from build123d import *

# Parameters (mm, degrees)
SKETCH1_W           = 90
SKETCH1_H           = 90
BOSS_EXTRUDE1_DEPTH = 70
SHELL2_T            = -5
CUT_EXTRUDE1_REACH  = 96.604
SKETCH2_W           = 70
SKETCH2_H           = 24
BOSS_EXTRUDE2_DEPTH = 7
SKETCH5_W           = 8
SKETCH5_H           = 10
CUT_EXTRUDE2_DEPTH  = 10


with BuildPart() as part:
    # Sketch1 → Boss-Extrude1 (new body)
    with BuildSketch(Plane.XY):
        Rectangle(SKETCH1_W, SKETCH1_H)
    extrude(amount=BOSS_EXTRUDE1_DEPTH)

    # Shell2
    shell2_openings = [part.faces().sort_by_distance(p)[0] for p in [
        (0, 0, 0),
    ]]
    offset(amount=SHELL2_T, openings=shell2_openings, kind=Kind.INTERSECTION)

    # Sketch2 → Cut-Extrude1 (cut, up to next)
    with BuildSketch(Plane.XY.offset(70), mode=Mode.PRIVATE) as cut_extrude1_sk1:
        with Locations((0, 20)):
            Rectangle(SKETCH2_W, SKETCH2_H)
    cut_extrude1_tool1 = extrude(cut_extrude1_sk1.sketch, amount=-CUT_EXTRUDE1_REACH, mode=Mode.PRIVATE) & part.part
    add(cut_extrude1_tool1.solids().sort_by_distance((0, 20, 70))[0], mode=Mode.SUBTRACT)

    # Sketch4 → Boss-Extrude2 (add)
    with BuildSketch(Plane(origin=(0, 0, 65), x_dir=(-1, 0, 0), z_dir=(0, 0, -1))):
        Polygon((-40, 38), (-40, 32), (-35, 32), (35, 32), (35, 8), (-35, 8), (-40, 8), (-40, 2), (40, 2), (40, 38), align=None)
    extrude(amount=BOSS_EXTRUDE2_DEPTH)

    # Sketch5 → Cut-Extrude2 (cut)
    with BuildSketch(Plane.XY.offset(70)):
        with Locations((0, -7)):
            Rectangle(SKETCH5_W, SKETCH5_H)
    extrude(amount=-CUT_EXTRUDE2_DEPTH, mode=Mode.SUBTRACT)


solid = part.part
Source: CAD feature listing. Evaluate the final solid. Frame: model axes, mm. A direction names the side the tool comes from. Round coordinates to 2 decimals unless told otherwise and drop trailing zeros. Loops run counter-clockwise (first coordinate to the right, second up) from the corner with the lowest first, then second, coordinate; pieces in that order, holes last. Notation, with made-up numbers: (74, 59) -> (114, 59) arc R13 ccw to (114, 66) -> close; hole circle Ø1 at (88, 24.5). An arc over 180 degrees is marked (long way). Answer as a JSON object with one key per item and string values. Group by question number.
Q1. Section query D-D (x = -2). Output: boundary loops of the cut face in (y, z), plus the area to 3 significant figures.
Q2. Contact query for a flat-ended pin moving along its axis: P1, Ø12.5, axis at x = -18, y = -21.5, coming from the -Z side. Output: stop coordinate, or through.
Q3. Access query for faces 5 (the flat face through (35, 20, 68)), 6 (the flat face through (-1, 40, 32)), 7 (the flat face through (-45, -1, 35)). Directions: +Z, -Z, +X, -X, +Y, -Y. A direction counts if a zero-diameter tool reaches every point of the face in a straight line with its end or side. Return the directions, or none.
Q4. Mould query, pull axis X, two halves, no side actions, for faces 1 (the flat face through (45, -1, 35)), 2 (the flat face through (0, -12, 68)), 3 (the flat face through (-1, 45, 35)), 4 (the flat face through (3, 32, 64)). Classes: pulls with the +X half, pulls with the -X half, needs draft (parallel to the pull), parting line crosses it, or undercut.
Q5. Section query C-C (z = 52.5). Output: boundary loops of the cut face in (x, y), plus the area to 3 significant figures.
Q6. Section query B-B (y = 10). Output: boundary loops of the cut face in (x, z).
Q7. Section query A-A (x = -20). Output: boundary loops of the cut face in (y, z).
Q8. Ray query, line 1 (X direction, y = 27, z = 50); line 2 (Z direction, x = 25.5, y = 0). Return the intervals inside material, ascending. Write a range as from..to.
Completed:
{
 "1": {"outline": "(-45, 0) -> (-40, 0) -> (-40, 65) -> (-12, 65) -> (-12, 70) -> (-45, 70) -> close; (-2, 65) -> (2, 65) -> (2, 58) -> (8, 58) -> (8, 70) -> (-2, 70) -> close; (32, 58) -> (38, 58) -> (38, 65) -> (40, 65) -> (40, 0) -> (45, 0) -> (45, 70) -> (32, 70) -> close", "area": "1,010 mm²"},
 "2": {"P1": "z = 65"},
 "3": {"face 5": "+Z, -Z", "face 6": "-Z", "face 7": "+Z, -Z, -X, +Y, -Y"},
 "4": {"face 1": "pulls with the +X half", "face 2": "undercut", "face 3": "needs draft", "face 4": "undercut"},
 "5": {"outline": "(-45, -45) -> (45, -45) -> (45, 45) -> (-45, 45) -> close; hole (-40, -40) -> (40, -40) -> (40, 40) -> (-40, 40) -> close", "area": "1,700 mm²"},
 "6": {"outline": "(-45, 0) -> (-40, 0) -> (-40, 58) -> (-35, 58) -> (-35, 70) -> (-45, 70) -> close; (35, 65) -> (40, 65) -> (40, 0) -> (45, 0) -> (45, 70) -> (35, 70) -> close"},
 "7": {"outline": "(-45, 0) -> (-40, 0) -> (-40, 65) -> (2, 65) -> (2, 58) -> (8, 58) -> (8, 70) -> (-45, 70) -> close; (32, 58) -> (38, 58) -> (38, 65) -> (40, 65) -> (40, 0) -> (45, 0) -> (45, 70) -> (32, 70) -> close"},
 "8": {"line 1": "-45..-40, 40..45", "line 2": "65..70"}
}
